The model under review builds one solid part; all positions refer to its coordinate system, in mm. A direction names the side the tool comes from. Coordinates: 2 decimals unless noted, no trailing zeros. Loops run counter-clockwise (first coordinate to the right, second up) from the corner with the lowest first, then second, coordinate; pieces in that order, holes last. Notation, with made-up numbers: M 63,-7.75 L 69,-7.75 A9 ccw 69,2.25 Z; hole C 52.25,12.25 d7. An arc over 180 degrees is marked long. Use CSV: the item, a comma, the result in double quotes. Start each with the question number.
1. Add section D-D, the plane z = -8.5. Write out the cut boundary in (x, y), then the cut area to 3 significant figures.
2. Tool access review of faces 5 (the flat face through (17, 8, -7.926)), 6 (the flat face through (-16.782, 8, -5)), 7 (the flat face through (9, 8, 0)): name each direction out of +Z, -Z, +X, -X, +Y, -Y from which nothing blocks a thin tool from reaching the whole face with its end or side.
3. Clearance check with flat-ended pins moving along their axes: P1, Ø0.6, axis at y = 10.5, z = -5.5, coming from the +X side; P2, Ø2, axis at x = 19.5, z = -9.5, coming from the +Y side; P3, Ø8, axis at x = 15.5, y = 13, coming from the -Z side; P4, Ø3.5, axis at x = -15, y = 6.5, coming from the -Z side. State where each tip first meets the part, or that it passes through.
4. Add section A-A, the plane y = 1.5. Write out the cut boundary in (x, z) (3 decimals), then the cut area to 3 significant figures.
5. Add section B-B, the plane x = 20.07. Write out the cut boundary in (y, z) (1 decimal).
6. Add section C-C, the plane y = 7. Write out the cut boundary in (x, z).
7. For L1, parallel to Z at x = 20.07, y = 12.85 (3 decimals); L2, parallel to Y at x = 16, z = 1; L3, parallel to Z at x = -4, y = 4, list the stretches that pass through material, from the lowest coordinate up.
8. Draft analysis for pull direction Y (two halves, no side actions). For faces 1 (the cylindrical face through (17.7, 7.676, -4.204)), 2 (the flat face through (2, 0, -5)), 3 (the flat face through (17.8, 11.62, -0.7)), 4 (the cylindrical face through (21.74, 1.78, 4.12)), state which applies: +Y half, -Y half, draft (parallel to the pull), parting line (faces both ways), or undercut.
from build123d import *

# Parameters (mm, degrees)
SKETCH1_R           = 2.2
BOSS_EXTRUDE1_DEPTH = 15.24
SKETCH2_R           = 4.826
CUT_EXTRUDE1_DEPTH  = 4.0005
FILLET2_R           = 2.54
FILLET3_R           = 2.54


with BuildPart() as part:
    # Sketch1 → Boss-Extrude1 (new body)
    with BuildSketch(Plane(origin=(0, 0, 0), x_dir=(1, 0, 0), z_dir=(0, 1, 0))):
        with BuildLine():
            Line((-19.782278513, 0), (-13.782278513, 0))
            Line((-13.782278513, 0), (-1.651, 0))
            ThreePointArc((-1.651, 0), (0, 1.651), (1.651, 0))
            Line((1.651, 0), (15.625, 0))
            ThreePointArc((15.625, 0), (22.30372167, -3.84298224), (22.27, 3.862385921))
            Line((22.27, 3.862385921), (22.27, 7.926385921))
            Line((22.27, 7.926385921), (11.963427905, 7.926385921))
            ThreePointArc((11.963427905, 7.926385921), (6.7896847, 12.64323466), (0, 14.351))
            ThreePointArc((0, 14.351), (-8.618213301, 11.475086078), (-13.782278513, 4))
            Line((-13.782278513, 4), (-16.782278513, 4))
            Line((-16.782278513, 4), (-16.782278513, 6))
            Line((-16.782278513, 6), (-19.782278513, 4))
            Line((-19.782278513, 4), (-19.782278513, 0))
        make_face()
        with Locations(Location((20.07, 0, 0), (0, 0, 90))):
            Circle(SKETCH1_R, mode=Mode.SUBTRACT)
    extrude(amount=BOSS_EXTRUDE1_DEPTH)

    # Sketch2 → Cut-Extrude1 (cut, symmetric)
    with BuildSketch(Plane(origin=(0, 7.62, 0), x_dir=(1, 0, 0), z_dir=(0, 1, 0))):
        with Locations((20.07, 0)):
            Circle(SKETCH2_R)
    extrude(amount=CUT_EXTRUDE1_DEPTH, both=True, mode=Mode.SUBTRACT)

    # Fillet2
    fillet2_edges = [part.edges().sort_by_distance(p)[0] for p in [
        (0, 15.24, -1.651),
    ]]
    fillet(fillet2_edges, radius=FILLET2_R)

    # Fillet3
    # the kernel refuses this fillet: 2.54 mm, written as the material it adds along each edge
    with BuildSketch(Plane(origin=(22.27, 4.011467753, -3.862385921), x_dir=(0.8069614715901079, 0, 0.5906040834341796), z_dir=(0, 1, 0))) as fillet3_piece_1_section:
        with BuildLine():
            CenterArc((1.300694552, 2.523500349), FILLET3_R, 216.19988752, 47.265895784)
            Line((-0.748987586, 1.023365977), (-0.789981229, 0.993363289))
            Line((-0.789981229, 0.993363289), (-0.040993643, -0.030002687))
            Line((-0.040993643, -0.030002687), (0.005780865, -0.050470007))
            ThreePointArc((0.005780865, -0.050470007), (0.505825659, -0.02192561), (1.005870453, -0.050470007))
            Line((1.005870453, -0.050470007), (1.011651318, 0))
        make_face()
    fillet3_piece_1 = extrude(amount=11.228532247, mode=Mode.PRIVATE)
    fillet3_piece_1 = split(fillet3_piece_1, bisect_by=Plane(origin=(22.284641862, 11.6205, -4.588750924), z_dir=(0, -1, 0)), keep=Keep.TOP, mode=Mode.PRIVATE)
    fillet3_piece_1 = fillet3_piece_1 - Plane(origin=(20.07, 7.815983876, 0), x_dir=(1, 0, 0), z_dir=(0, 1, 0)) * Cylinder(4.826, 27, mode=Mode.PRIVATE)
    add(fillet3_piece_1)
    with BuildSketch(Plane(origin=(22.27, 11.6205, -3.862385921), x_dir=(0.8069614715901079, 0, 0.5906040834341796), z_dir=(0, 1, 0))) as fillet3_piece_2_section:
        with BuildLine():
            CenterArc((1.300694552, 2.523500349), FILLET3_R, 216.19988752, 47.265895784)
            Line((-0.748987586, 1.023365977), (-0.789981229, 0.993363289))
            Line((-0.789981229, 0.993363289), (-0.040993643, -0.030002687))
            Line((-0.040993643, -0.030002687), (0.005780865, -0.050470007))
            ThreePointArc((0.005780865, -0.050470007), (0.505825659, -0.02192561), (1.005870453, -0.050470007))
            Line((1.005870453, -0.050470007), (1.011651318, 0))
        make_face()
    fillet3_piece_2 = extrude(amount=3.6195, mode=Mode.PRIVATE)
    fillet3_piece_2 = fillet3_piece_2 & Plane(origin=(20.07, 13.43025, 0), x_dir=(1, 0, 0), z_dir=(0, 1, 0)) * Cylinder(4.826, 12, mode=Mode.PRIVATE)
    add(fillet3_piece_2)
    with BuildSketch(Plane(origin=(22.27, 11.6205, -3.862385921), x_dir=(0.8069614715901079, 0, 0.5906040834341796), z_dir=(0, 1, 0))) as fillet3_piece_3_section:
        with BuildLine():
            CenterArc((1.300694552, 2.523500349), FILLET3_R, 216.19988752, 47.265895784)
            Line((-0.748987586, 1.023365977), (-0.789981229, 0.993363289))
            Line((-0.789981229, 0.993363289), (-0.040993643, -0.030002687))
            Line((-0.040993643, -0.030002687), (0.005780865, -0.050470007))
            ThreePointArc((0.005780865, -0.050470007), (0.505825659, -0.02192561), (1.005870453, -0.050470007))
            Line((1.005870453, -0.050470007), (1.011651318, 0))
        make_face()
    fillet3_piece_3 = extrude(amount=3.6195, mode=Mode.PRIVATE)
    fillet3_piece_3 = fillet3_piece_3 - Plane(origin=(20.07, 13.43025, 0), x_dir=(1, 0, 0), z_dir=(0, 1, 0)) * Cylinder(4.826, 12, mode=Mode.PRIVATE)
    add(fillet3_piece_3)
    with BuildSketch(Plane(origin=(22.27, 0, -3.862385921), x_dir=(0, 0, -1), z_dir=(0, 1, 0))) as fillet3_piece_4_section:
        with BuildLine():
            CenterArc((1.268172041, -2.54), FILLET3_R, 90, 47.265895784)
            Line((-0.597485399, -0.816363636), (-0.634798548, -0.781890909))
            ThreePointArc((-0.634798548, -0.781890909), (-0.316435822, -0.395232463), (-0.044141553, 0.025142857))
            Line((-0.044141553, 0.025142857), (0, 0.0508))
            Line((0, 0.0508), (1.268172041, 0.0508))
            Line((1.268172041, 0.0508), (1.268172041, 0))
        make_face()
    fillet3_piece_4 = extrude(amount=3.6195, mode=Mode.PRIVATE)
    fillet3_piece_4 = fillet3_piece_4 - Plane(origin=(20.07, 1.80975, 0), x_dir=(1, 0, 0), z_dir=(0, 1, 0)) * Cylinder(4.826, 13, mode=Mode.PRIVATE)
    add(fillet3_piece_4)
    with BuildSketch(Plane(origin=(22.27, 0, -3.862385921), x_dir=(0, 0, -1), z_dir=(0, 1, 0))) as fillet3_piece_5_section:
        with BuildLine():
            CenterArc((1.268172041, -2.54), FILLET3_R, 90, 47.265895784)
            Line((-0.597485399, -0.816363636), (-0.634798548, -0.781890909))
            ThreePointArc((-0.634798548, -0.781890909), (-0.316435822, -0.395232463), (-0.044141553, 0.025142857))
            Line((-0.044141553, 0.025142857), (0, 0.0508))
            Line((0, 0.0508), (1.268172041, 0.0508))
            Line((1.268172041, 0.0508), (1.268172041, 0))
        make_face()
    fillet3_piece_5 = extrude(amount=3.6195, mode=Mode.PRIVATE)
    fillet3_piece_5 = fillet3_piece_5 & Plane(origin=(20.07, 1.80975, 0), x_dir=(1, 0, 0), z_dir=(0, 1, 0)) * Cylinder(4.826, 13, mode=Mode.PRIVATE)
    add(fillet3_piece_5)
    with BuildSketch(Plane(origin=(22.27, 0, -3.862385921), x_dir=(0, 0, -1), z_dir=(0, 1, 0))) as fillet3_piece_6_section:
        with BuildLine():
            CenterArc((1.268172041, -2.54), FILLET3_R, 90, 47.265895784)
            Line((-0.597485399, -0.816363636), (-0.634798548, -0.781890909))
            ThreePointArc((-0.634798548, -0.781890909), (-0.316435822, -0.395232463), (-0.044141553, 0.025142857))
            Line((-0.044141553, 0.025142857), (0, 0.0508))
            Line((0, 0.0508), (1.268172041, 0.0508))
            Line((1.268172041, 0.0508), (1.268172041, 0))
        make_face()
    fillet3_piece_6 = extrude(amount=11.228532247, mode=Mode.PRIVATE)
    fillet3_piece_6 = fillet3_piece_6 - Plane(origin=(20.07, 7.424016124, 0), x_dir=(1, 0, 0), z_dir=(0, 1, 0)) * Cylinder(4.826, 28, mode=Mode.PRIVATE)
    fillet3_piece_6 = split(fillet3_piece_6, bisect_by=Plane(origin=(22.284641862, 3.6195, -4.588750924), z_dir=(0, 1, 0)), keep=Keep.TOP, mode=Mode.PRIVATE)
    add(fillet3_piece_6)


solid = part.part
Computed:
1,outline,"M -11.56,0 L 11.56,0 L 11.56,15.24 L -11.56,15.24 Z"
1,area,"352 mm^2"
2,face 5,"-Z, +X, +Y, -Y"
2,face 6,"-Z, +Y, -Y"
2,face 7,"+Z, -X, +Y, -Y"
3,P1,"stops at x = 22.27"
3,P2,"passes through"
3,P3,"stops at z = -8.58"
3,P4,"stops at z = -5.51"
4,outline,"M -19.782,-4 L -16.782,-6 L -16.782,-4 L -13.782,-4 A14.351 ccw 11.963,-7.926 L 22.27,-7.926 L 22.27,-5.131 A2.54 cw 23.086,-3.265 A4.445 ccw long 15.625,0 L 1.651,0 A1.651 cw -1.651,0 L -19.782,0 Z; hole C 20.07,0 d4.4"
4,area,"436 mm^2"
5,outline,"M 0,-7.9 L 15.2,-7.9 L 15.2,-2.2 L 11.6,-2.2 L 11.6,-4.8 L 3.6,-4.8 L 3.6,-2.2 L 0,-2.2 Z; M 0,2.2 L 3.6,2.2 L 3.6,4.4 L 0,4.4 Z; M 11.6,2.2 L 15.2,2.2 L 15.2,4.4 L 11.6,4.4 Z"
6,outline,"M -19.78,-4 L -16.78,-6 L -16.78,-4 L -13.78,-4 A14.35 ccw 11.96,-7.93 L 22.27,-7.93 L 22.27,-5.13 A2.54 cw 22.45,-4.2 A4.83 cw 15.24,0 L 1.65,0 A1.65 cw -1.65,0 L -19.78,0 Z"
7,L1,"z = -7.926 to -2.2, 2.2 to 4.445"
7,L2,"y = 0 to 3.62, 11.62 to 15.24"
7,L3,"z = -13.78 to 0"
8,face 1,"undercut"
8,face 2,"-Y half"
8,face 3,"undercut"
8,face 4,"draft"
